Answer from the drawing. Dimensions are ordinates in mm from the lowest x, y and z of the part. A direction names the side the tool comes from. Round coordinates to 2 decimals unless told otherwise and drop trailing zeros. Order: outer loops, then holes, each group sorted by start corner. A loop starts at its lowest first (then second) coordinate and runs counter-clockwise, first axis right, second up. Notation, with made-up numbers: (83, 81.25) -> (121, 81.25) arc R26 ccw to (121, 117.25) -> close; hole circle Ø2 at (-13.5, 32.25). An arc over 180 degrees is marked (long way). Use a Markdown table: item, result. Add a question column.
1. Section A-A, the plane y = 16 is taken. Give the vertices of the cut face in (x, z) (3 decimals), then the cut area to 3 significant figures.
2. Section C-C, the plane z = 15.5 is taken. Give the vertices of the cut face in (x, y).
3. Section D-D, the plane z = 6.75 is taken. Give the vertices of the cut face in (x, y).
4. Consider L1, parallel to Y at x = 16, z = 2; L2, parallel to X at y = 20.5, z = 13.5; L3, parallel to X at y = 21, z = 20.5. Determine where each line is inside the solid, lowest interval first. Write a range as [from, to].
5. Given pin 1 (2 mm diameter, centred on y = 16, z = 21, fed in from -X); pin 2 (6 mm diameter, centred on x = 7.5, z = 15.5, fed in from -Y); pin 3 (12 mm diameter, centred on y = 21, z = 18.5, fed in from +X), each flat-ended and moving along its own axis, determine where each tip first touches the part or whether it passes through.
6. For the marked faces 1 and 2, determine the directions among +Z, -Z, +X, -X, +Y, -Y from which every point of the face is accessible in a straight line to the end or side of a thin tool.
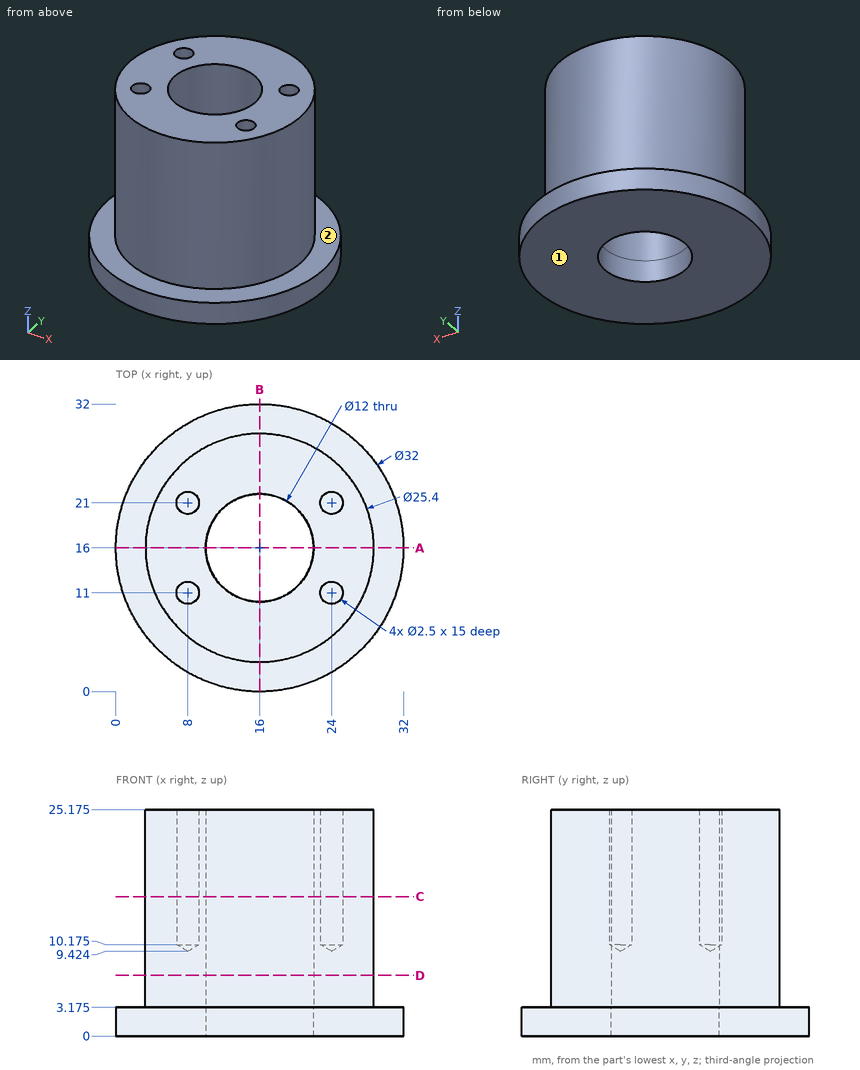
Verdict:
| question | item | result |
|---|---|---|
| 1 | outline | (0, 0) -> (10, 0) -> (10, 25.175) -> (3.3, 25.175) -> (3.3, 3.175) -> (0, 3.175) -> close; (22, 0) -> (32, 0) -> (32, 3.175) -> (28.7, 3.175) -> (28.7, 25.175) -> (22, 25.175) -> close |
| 1 | area | 358 mm2 |
| 2 | outline | circle Ø25.4 at (16, 16); hole circle Ø2.5 at (8, 11); hole circle Ø2.5 at (8, 21); hole circle Ø12 at (16, 16); hole circle Ø2.5 at (24, 11); hole circle Ø2.5 at (24, 21) |
| 3 | outline | circle Ø25.4 at (16, 16); hole circle Ø12 at (16, 16) |
| 4 | L1 | y = [0, 10], [22, 32] |
| 4 | L2 | x = [4.12, 6.85], [9.15, 12.03], [19.97, 22.85], [25.15, 27.88] |
| 4 | L3 | x = [4.33, 6.75], [9.25, 12.68], [19.32, 22.75], [25.25, 27.67] |
| 5 | pin 1 | stops at x = 3.3 |
| 5 | pin 2 | stops at y = 4.55 |
| 5 | pin 3 | stops at x = 28.7 |
| 6 | face 1 | -Z, +X, -X, +Y, -Y |
| 6 | face 2 | +Z |
